```python
from build123d import *

# Parameters (mm, degrees)
ESBO_O1_W                           = 76
ESBO_O1_H                           = 50
ESBO_O1_R                           = 2.5
ESBO_O1_R_2                         = 6
RESSALTO_EXTRUS_O1_DEPTH            = 3
ESBO_O2_R                           = 2.5
CORTE_EXTRUS_O1_DEPTH               = 3
FILETE1_R                           = 20
ESBO_O3_R                           = 1.5
CORTE_EXTRUS_O2_DEPTH               = 4
ESBO_O4_R                           = 2.5
ESBO_O4_R_2                         = 3
CORTE_EXTRUS_O3_DEPTH               = 4
RESSALTO_EXTRUS_O2_DEPTH            = 3
ESBO_O6_R                           = 3
RESSALTO_EXTRUS_O3_DEPTH            = 3
CORTE_EXTRUS_O4_DEPTH               = 4
CHANFRO1_SIZE                       = 1.5
ESCAREADO_PARA_SFHCS_M54_AT_2_COUNT = 2
ESCAREADO_PARA_SFHCS_M54_AT_2_PITCH = 25


with BuildPart() as part:
    # Esboço1 → Ressalto-extrusão1 (new body)
    with BuildSketch(Plane.XY):
        with Locations((38, 25)):
            Rectangle(ESBO_O1_W, ESBO_O1_H)
        with Locations((59.25, 18.5)):
            Circle(ESBO_O1_R, mode=Mode.SUBTRACT)
        with Locations((25, 25)):
            Circle(ESBO_O1_R_2, mode=Mode.SUBTRACT)
    extrude(amount=RESSALTO_EXTRUS_O1_DEPTH)

    # Esboço2 → Corte-extrusão1 (cut)
    with BuildSketch(Plane.XY.offset(3)):
        with Locations((66, 35)):
            Circle(ESBO_O2_R)
        with Locations((66, 10)):
            Circle(ESBO_O2_R)
    extrude(amount=-CORTE_EXTRUS_O1_DEPTH, mode=Mode.SUBTRACT)

    # Filete1
    filete1_edges = [part.edges().sort_by_distance(p)[0] for p in [
        (0, 50, 1.5),
        (0, 0, 1.5),
    ]]
    fillet(filete1_edges, radius=FILETE1_R)

    # Esboço3 → Corte-extrusão2 (cut, through all)
    with BuildSketch(Plane.XY.offset(3)):
        with Locations((33, 35)):
            Circle(ESBO_O3_R)
        with Locations((33, 15)):
            Circle(ESBO_O3_R)
        with Locations((17, 15)):
            Circle(ESBO_O3_R)
        with Locations((17, 35)):
            Circle(ESBO_O3_R)
    extrude(amount=-CORTE_EXTRUS_O2_DEPTH, mode=Mode.SUBTRACT)

    # Esboço4 → Corte-extrusão3 (cut, through all)
    with BuildSketch(Plane.XY.offset(3)):
        with Locations((45.680731562, 3.807316308)):
            Circle(ESBO_O4_R)
        with Locations((52.0071049, 37.142437356)):
            Circle(ESBO_O4_R_2)
    extrude(amount=-CORTE_EXTRUS_O3_DEPTH, mode=Mode.SUBTRACT)

    # Esboço5 → Ressalto-extrusão2 (add, through all)
    with BuildSketch(Plane(origin=(0, 0, 0), x_dir=(-1, 0, 0), z_dir=(0, 0, -1))):
        with BuildLine():
            Line((-20, 0), (-76, 0))
            Line((-76, 0), (-46.796939635, -4.11469761))
            ThreePointArc((-46.796939635, -4.11469761), (-45.615731629, -4.192683692), (-44.435946758, -4.095514563))
            Line((-44.435946758, -4.095514563), (-16.888140703, 0.243574926))
            ThreePointArc((-16.888140703, 0.243574926), (-18.439311288, 0.060986716), (-20, 0))
        make_face()
    extrude(amount=-RESSALTO_EXTRUS_O2_DEPTH)

    # Esboço6 → Ressalto-extrusão3 (add, through all)
    with BuildSketch(Plane(origin=(0, 0, 0), x_dir=(-1, 0, 0), z_dir=(0, 0, -1))):
        with BuildLine():
            ThreePointArc((-88.7, 21.731512949), (-88.256556331, 18.786647741), (-86.965553781, 16.102958899))
            Line((-86.965553781, 16.102958899), (-78.060298944, 3.02555711))
            ThreePointArc((-78.060298944, 3.02555711), (-77.114291558, 1.840577528), (-76, 0.812248345))
            Line((-76, 0.812248345), (-76, 48.486996415))
            ThreePointArc((-76, 48.486996415), (-77.637464746, 47.21301111), (-78.976802336, 45.628554049))
            Line((-78.976802336, 45.628554049), (-86.965553781, 33.897041101))
            ThreePointArc((-86.965553781, 33.897041101), (-88.256556331, 31.213352259), (-88.7, 28.268487051))
            Line((-88.7, 28.268487051), (-88.7, 21.731512949))
        make_face()
        with Locations((-82.35, 25)):
            Circle(ESBO_O6_R, mode=Mode.SUBTRACT)
    extrude(amount=-RESSALTO_EXTRUS_O3_DEPTH)

    # Esboço7 → Corte-extrusão4 (cut, through all)
    with BuildSketch(Plane(origin=(0, 0, 0), x_dir=(-1, 0, 0), z_dir=(0, 0, -1))):
        with BuildLine():
            ThreePointArc((-78.060298944, 3.02555711), (-77.114291558, 1.840577528), (-76, 0.812248345))
            Line((-76, 0.812248345), (-76, 0))
            Line((-76, 0), (-72.447166346, -0.500592608))
            ThreePointArc((-72.447166346, -0.500592608), (-75.585868949, 0.73376814), (-78.060298944, 3.02555711))
        make_face()
        with BuildLine():
            Line((-76, 50), (-76, 48.486996415))
            ThreePointArc((-76, 48.486996415), (-73.461706321, 49.614311316), (-70.711248555, 50))
            Line((-70.711248555, 50), (-76, 50))
        make_face()
    extrude(amount=-CORTE_EXTRUS_O4_DEPTH, mode=Mode.SUBTRACT)

    # Chanfro1
    chanfro1_edges = [part.edges().sort_by_distance(p)[0] for p in [
        (15.5, 35, 0),
        (15.5, 15, 0),
        (31.5, 15, 0),
        (31.5, 35, 0),
    ]]
    chamfer(chanfro1_edges, length=CHANFRO1_SIZE)

    # Esboço17 → Escareado para SFHCS M51 (revolve, cut)
    with BuildSketch(Plane(origin=(45.680731562, 3.807316308, 3), x_dir=(0, -1, 0), z_dir=(1, 0, 0))):
        Polygon((0, 0), (0, 3), (2.75, 3), (2.75, 2.85), (5.6, 0), align=None)
    revolve(axis=Axis((45.680731562, 3.807316308, 9.35), (0, 0, -1)), mode=Mode.SUBTRACT)

    # Esboço19 → Escareado para SFHCS M52 (revolve, cut)
    with BuildSketch(Plane(origin=(59.25, 18.5, 3), x_dir=(0, -1, 0), z_dir=(1, 0, 0))):
        Polygon((0, 0), (0, 3), (2.75, 3), (2.75, 2.85), (5.6, 0), align=None)
    revolve(axis=Axis((59.25, 18.5, 9.35), (0, 0, -1)), mode=Mode.SUBTRACT)

    # Esboço23 → Escareado para SFHCS M54 (revolve, cut)
    with BuildSketch(Plane(origin=(66, 35, 0), x_dir=(0, 1, 0), z_dir=(1, 0, 0))):
        Polygon((0, 0), (0, 3), (2.75, 3), (2.75, 2.85), (5.6, 0), align=None)
    escareado_para_sfhcs_m54 = revolve(axis=Axis((66, 35, -6.35), (0, 0, 1)), mode=Mode.SUBTRACT)

    # Escareado para SFHCS M54 at 2: Escareado para SFHCS M54 ×2
    with Locations(*[(0, -i * ESCAREADO_PARA_SFHCS_M54_AT_2_PITCH, 0) for i in range(1, ESCAREADO_PARA_SFHCS_M54_AT_2_COUNT)]):
        add(escareado_para_sfhcs_m54, mode=Mode.SUBTRACT)


solid = part.part
```
Could you check a few things on this model? Use its own coordinates, in mm. Round coordinates to 2 decimals unless told otherwise and drop trailing zeros. Loops run counter-clockwise (first coordinate to the right, second up) from the corner with the lowest first, then second, coordinate; pieces in that order, holes last. Notation, with made-up numbers: M 29,-31 L 46,-31 A14 ccw 46,-27 Z; hole C 73.5,-36.5 d2. An arc over 180 degrees is marked long. Answer as CSV lines item,"result".
1) Imagine slicing it at D-D on x = 66. List the corners of the cut face in (y, z) for me, and give its area (3 significant figures).
From the geometry:
outline,"M -1.41,0 L 4.4,0 L 7.25,2.85 L 7.25,3 L -1.41,3 Z; M 12.75,2.85 L 15.6,0 L 29.4,0 L 32.25,2.85 L 32.25,3 L 12.75,3 Z; M 37.75,2.85 L 40.6,0 L 50,0 L 50,3 L 37.75,3 Z"
area,"105 mm^2"
2) Imagine slicing it at C-C on x = 81. List the corners of the cut face in (y, z) for me, and give its area (3 significant figures).
From the geometry:
outline,"M 7.34,0 L 22.32,0 L 22.32,3 L 7.34,3 Z; M 27.68,0 L 42.66,0 L 42.66,3 L 27.68,3 Z"
area,"89.9 mm^2"
3) We'd pull the mould along X, two halves only. Please class faces 1 (the cylindrical face through (31.5, 15.07, 2.26)), 2 (the cylindrical face through (5.703, 43.986, 1.521)), 3 (the cylindrical face through (88.27, 18.83, 1.48)): released by +X, released by -X, zero draft, split by the parting line, or undercut.
From the geometry:
face 1,"undercut"
face 2,"released by -X"
face 3,"released by +X"
4) Imagine slicing it at A-A on x = 33. List the corners of the cut face in (y, z) for me, and give its area (3 significant figures).
From the geometry:
outline,"M -2.29,0 L 12,0 L 13.5,1.5 L 13.5,3 L -2.29,3 Z; M 16.5,1.5 L 18,0 L 32,0 L 33.5,1.5 L 33.5,3 L 16.5,3 Z; M 36.5,1.5 L 38,0 L 50,0 L 50,3 L 36.5,3 Z"
area,"134 mm^2"
5) For pin 1 Ø6.5 at (x, y) = (45.68, 3.81) entering from -Z; pin 2 Ø1.5 at (x, z) = (29.5, 1) entering from -Y; pin 3 Ø9 at (x, y) = (66, 10) entering from -Z; pin 4 Ø3.5 at (x, y) = (17, 35) entering from -Z, each with a flat end and sliding along its axis, tell me the tip position at first contact or that it passes through.
From the geometry:
pin 1,"z = 0"
pin 2,"y = -1.86"
pin 3,"z = 1.1"
pin 4,"z = 1.25"
6) Imagine slicing it at B-B on x = 52.5. List the corners of the cut face in (y, z) for me.
From the geometry:
outline,"M -3.31,0 L 34.18,0 L 34.18,3 L -3.31,3 Z; M 40.1,0 L 50,0 L 50,3 L 40.1,3 Z"
7) If I drill on probe 1 along Y at (x, z) = (33, 1.95); probe 2 along X at (y, z) = (37.5, 2.4); probe 3 along Y at (x, z) = (17, 1.95), over which ranges is the centre line in solid material (lowest first)?
From the geometry:
probe 1,"-2.29 to 13.5, 16.5 to 33.5, 36.5 to 50"
probe 2,"1.46 to 49.03, 54.99 to 64, 68 to 84.51"
probe 3,"0.23 to 13.5, 16.5 to 33.5, 36.5 to 49.77"
